Geometry check sheet. Reference: the model listing, model coordinates, mm. Face numbers are marked on the shaded views. A direction names the side the tool comes from. Coordinates: 2 decimals unless noted, no trailing zeros. Loops run counter-clockwise (first coordinate to the right, second up) from the corner with the lowest first, then second, coordinate; pieces in that order, holes last.
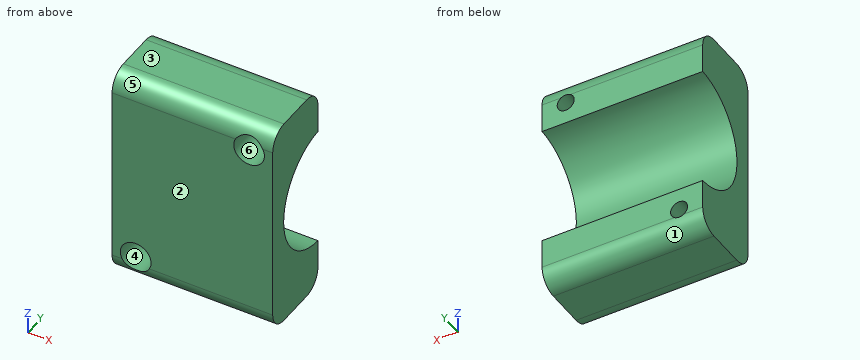
from build123d import *

# Parameters (mm, degrees)
BOSS_EXTRUDE1_DEPTH     = 17
CUT_EXTRUDE1_DEPTH      = 34.119329703
CUT_EXTRUDE1_DEPTH_BACK = 34.119329703
SKETCH2_R               = 12.8
SKETCH3_R               = 1.8
CUT_EXTRUDE2_DEPTH      = 17
SKETCH4_R               = 3.25
CUT_EXTRUDE3_DEPTH      = 7.5


with BuildPart() as part:
    # Sketch1 → Boss-Extrude1 (new, symmetric)
    with BuildSketch(Plane(origin=(0, 0, 0), x_dir=(0, 0, -1), z_dir=(1, 0, 0))):
        with BuildLine():
            Line((-19, -16.7), (19, -16.7))
            ThreePointArc((19, -16.7), (21.828427125, -15.528427125), (23, -12.7))
            Line((23, -12.7), (23, -4.6))
            ThreePointArc((23, -4.6), (21.828427125, -1.771572875), (19, -0.6))
            Line((19, -0.6), (-19, -0.6))
            ThreePointArc((-19, -0.6), (-21.828427125, -1.771572875), (-23, -4.6))
            Line((-23, -4.6), (-23, -12.7))
            ThreePointArc((-23, -12.7), (-21.828427125, -15.528427125), (-19, -16.7))
        make_face()
    extrude(amount=BOSS_EXTRUDE1_DEPTH, both=True)

    # Sketch2 → Cut-Extrude1 (cut, two sides: drawn at the far end of the back side and taken through both)
    with BuildSketch(Plane(origin=(0, 0, 0), x_dir=(0, 0, -1), z_dir=(1, 0, 0)).offset(-CUT_EXTRUDE1_DEPTH_BACK)):
        Circle(SKETCH2_R)
    extrude(amount=CUT_EXTRUDE1_DEPTH + CUT_EXTRUDE1_DEPTH_BACK, mode=Mode.SUBTRACT)

    # Sketch3 → Cut-Extrude2 (cut)
    with BuildSketch(Plane(origin=(0, -16.7, 0), x_dir=(1, 0, 0), z_dir=(0, 1, 0))):
        with Locations(Location((12, -17.5, 0), (0, 0, 236.442690238))):
            Circle(SKETCH3_R)
        with Locations(Location((-12, 17.5, 0), (0, 0, 56.442690238))):
            Circle(SKETCH3_R)
    extrude(amount=CUT_EXTRUDE2_DEPTH, mode=Mode.SUBTRACT)

    # Sketch4 → Cut-Extrude3 (cut)
    with BuildSketch(Plane(origin=(0, -16.7, 0), x_dir=(1, 0, 0), z_dir=(0, 1, 0))):
        with Locations(Location((12, -17.5, 0), (0, 0, 207.48642625))):
            Circle(SKETCH4_R)
        with Locations(Location((-12, 17.5, 0), (0, 0, 27.48642625))):
            Circle(SKETCH4_R)
    extrude(amount=CUT_EXTRUDE3_DEPTH, mode=Mode.SUBTRACT)


solid = part.part
(1) Sectioned sample at D-D on y = -2.25. Record the cut outline in (x, z).
Findings:
outline: (-17, -22.24) - (17, -22.24) - (17, -12.6) - (-17, -12.6) - close; (-17, 12.6) - (17, 12.6) - (17, 22.24) - (-17, 22.24) - close; hole circle Ø3.6 at (-12, -17.5); hole circle Ø3.6 at (12, 17.5)
(2) Sectioned sample at A-A on y = -6.75. Record the cut outline in (x, z).
Findings:
outline: (-17, -23) - (17, -23) - (17, -10.88) - (-17, -10.88) - close; (-17, 10.88) - (17, 10.88) - (17, 23) - (-17, 23) - close; hole circle Ø3.6 at (-12, -17.5); hole circle Ø3.6 at (12, 17.5)
(3) Gauge pin test, flat ends, axial feed: pin 1 Ø10.5 at (x, z) = (12, 17.5) entering from +Y; pin 2 Ø4 at (x, z) = (-12, -17.5) entering from -Y. Record the tip position at first contact, or that the pin passes through.
Findings:
pin 1: stops at y = -0.6
pin 2: stops at y = -9.2
(4) Access from +Z, -Z, +X, -X, +Y, -Y to the whole of each face (thin tool, end or side, straight path). Record for the marked faces 5 and 6.
Findings:
face 5: +Z, +X, -X, -Y
face 6: -Y
(5) Scan lines: L1, parallel to X at y = -12, z = -17.5; L2, parallel to X at y = -5.25, z = 17.5; L3, parallel to Z at x = -12, y = -4. Record each from-to range of solid material in increasing order.
Findings:
L1: x = -17 to -15.25, -8.75 to 17
L2: x = -17 to 10.2, 13.8 to 17
L3: z = -22.95 to -19.3, -15.7 to -12.16, 12.16 to 22.95
(6) Sectioned sample at C-C on x = 12. Record the cut outline in (y, z), and give its area (3 significant figures).
Findings:
outline: (-16.7, -19) arc R4 ccw to (-12.7, -23) - (-4.6, -23) arc R4 ccw to (-0.6, -19) - (-0.6, -12.79) arc R12.8 cw to (-0.6, 12.79) - (-0.6, 15.7) - (-9.2, 15.7) - (-9.2, 14.25) - (-16.7, 14.25) - close; (-16.3, 20.75) - (-9.2, 20.75) - (-9.2, 19.3) - (-0.61, 19.3) arc R4 ccw to (-4.6, 23) - (-12.7, 23) arc R4 ccw to start
area: 405 mm2
(7) Sectioned sample at B-B on z = 17.5. Record the cut outline in (x, y), and give its area (3 significant figures).
Findings:
outline: (-17, -16.7) - (8.75, -16.7) - (8.75, -9.2) - (10.2, -9.2) - (10.2, -0.6) - (-17, -0.6) - close; (13.8, -9.2) - (15.25, -9.2) - (15.25, -16.7) - (17, -16.7) - (17, -0.6) - (13.8, -0.6) - close
area: 468 mm2
(8) Draft check along Z on the marked faces 1, 2, 3 and 4. Enter one of: +Z half, -Z half, draft (parallel to the pull), parting line (faces both ways), or undercut.
Findings:
face 1: -Z half
face 2: draft
face 3: +Z half
face 4: undercut
